The model under review builds one solid part; all positions refer to its coordinate system, in mm. Face numbers are marked on the shaded views. A direction names the side the tool comes from. Coordinates: 2 decimals unless noted, no trailing zeros. Write each loop counter-clockwise with the first axis right and the second up, starting at its lowest first coordinate (ties: lowest second). Pieces come first, ordered by that corner, then holes. Notation, with made-up numbers: (-10, -29.5) - (5, -29.5) arc R5 ccw to (5, -24.5) - close; hole circle Ø1 at (27.5, 3). An arc over 180 degrees is marked (long way). Return JSON: item names as keys, results as strings. Group by question number.
(1) For pin 1 Ø3.5 at (x, y) = (13.5, 9.5) entering from +Z; pin 2 Ø8 at (x, y) = (-14, -9.5) entering from -Z; pin 3 Ø8 at (x, y) = (0.5, 6.5) entering from +Z, all flat-tipped, find the tip position at first contact; note any pin that passes through.
(2) We need section A-A on z = 10.5. State the section outline as (x, y) points.
(3) Draft analysis for pull direction X (two halves, no side actions). For the marked faces 1, 2 and 3, state which applies: released by +X, released by -X, zero draft, split by the parting line, or undercut.
(4) We need section C-C on x = 13. State the section outline as (y, z) points.
(5) To check wall thickness, follow L1, parallel to Y at x = -13, z = 9.5; L2, parallel to Y at x = -15, z = 8; L3, parallel to X at y = -12.5, z = 13.25. State the ranges of each line that lie inside material, in increasing order. Write a range as from..to.
(6) We need section D-D on y = -4. State the section outline as (x, z) points.
(7) We need section B-B on z = 14.25. State the section outline as (x, y) points.
(8) Tool access review of the marked faces 4 and 5: name each direction out of +Z, -Z, +X, -X, +Y, -Y from which nothing blocks a thin tool from reaching the whole face with its end or side.
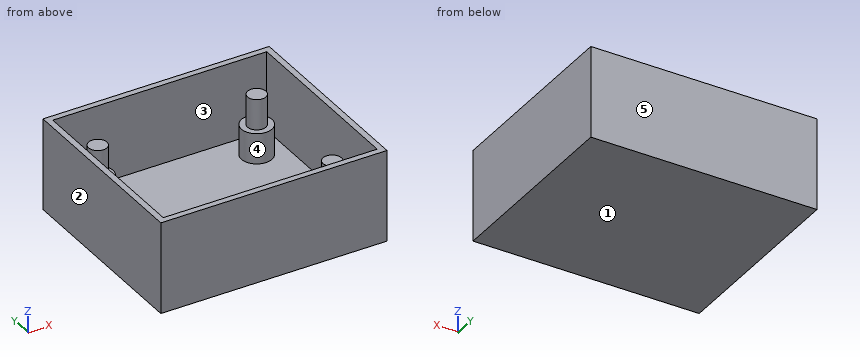
```python
from build123d import *

# Parameters (mm, degrees)
F1_W     = 37
F1_H     = 32
F2_DEPTH = 15
F3_W     = 35
F3_H     = 30
F4_DEPTH = 13
F5_R     = 2.5
F5_R_2   = 1.5
F6_DEPTH = 5
F7_DEPTH = 10


with BuildPart() as f2:
    # F1 (on Top) → F2 (new body)
    with BuildSketch(Plane.XY):
        Rectangle(F1_W, F1_H)
    extrude(amount=F2_DEPTH)

    # F3 (on face) → F4 (cut)
    with BuildSketch(Plane.XY.offset(15)):
        Rectangle(F3_W, F3_H)
    extrude(amount=-F4_DEPTH, mode=Mode.SUBTRACT)

    # F5 (on face) → F6 (join)
    with BuildSketch(Plane.XY.offset(2)):
        with Locations((-13, 10.25)):
            Circle(F5_R)
        with Locations((-13, 10.25)):
            Circle(F5_R_2, mode=Mode.SUBTRACT)
        with Locations((13, 10.25)):
            Circle(F5_R)
        with Locations((13, 10.25)):
            Circle(F5_R_2, mode=Mode.SUBTRACT)
        with Locations((13, -10.25)):
            Circle(F5_R)
        with Locations((13, -10.25)):
            Circle(F5_R_2, mode=Mode.SUBTRACT)
        with Locations((-13, 10.25)):
            Circle(F5_R_2)
        with Locations((13, 10.25)):
            Circle(F5_R_2)
        with Locations((13, -10.25)):
            Circle(F5_R_2)
    extrude(amount=F6_DEPTH)

    # F5 (on face) → F7 (join)
    with BuildSketch(Plane.XY.offset(2)):
        with Locations((-13, 10.25)):
            Circle(F5_R_2)
        with Locations((13, 10.25)):
            Circle(F5_R_2)
        with Locations((13, -10.25)):
            Circle(F5_R_2)
    extrude(amount=F7_DEPTH)


solid = f2.part
```
Ans:
{
 "1": {"pin 1": "z = 12", "pin 2": "z = 0", "pin 3": "z = 2"},
 "2": {"outline": "(-18.5, -16) - (18.5, -16) - (18.5, 16) - (-18.5, 16) - close; circle Ø3 at (-13, 10.25); circle Ø3 at (13, -10.25); circle Ø3 at (13, 10.25); hole (-17.5, -15) - (17.5, -15) - (17.5, 15) - (-17.5, 15) - close"},
 "3": {"face 1": "zero draft", "face 2": "released by -X", "face 3": "undercut"},
 "4": {"outline": "(-16, 0) - (16, 0) - (16, 15) - (15, 15) - (15, 2) - (12.75, 2) - (12.75, 7) - (11.75, 7) - (11.75, 12) - (8.75, 12) - (8.75, 7) - (7.75, 7) - (7.75, 2) - (-7.75, 2) - (-7.75, 7) - (-8.75, 7) - (-8.75, 12) - (-11.75, 12) - (-11.75, 7) - (-12.75, 7) - (-12.75, 2) - (-15, 2) - (-15, 15) - (-16, 15) - close"},
 "5": {"L1": "-16..-15, 8.75..11.75, 15..16", "L2": "-16..-15, 15..16", "L3": "-18.5..-17.5, 17.5..18.5"},
 "6": {"outline": "(-18.5, 0) - (18.5, 0) - (18.5, 15) - (17.5, 15) - (17.5, 2) - (-17.5, 2) - (-17.5, 15) - (-18.5, 15) - close"},
 "7": {"outline": "(-18.5, -16) - (18.5, -16) - (18.5, 16) - (-18.5, 16) - close; hole (-17.5, -15) - (17.5, -15) - (17.5, 15) - (-17.5, 15) - close"},
 "8": {"face 4": "+Z", "face 5": "+Z, -Z, +X, -X, +Y"}
}
